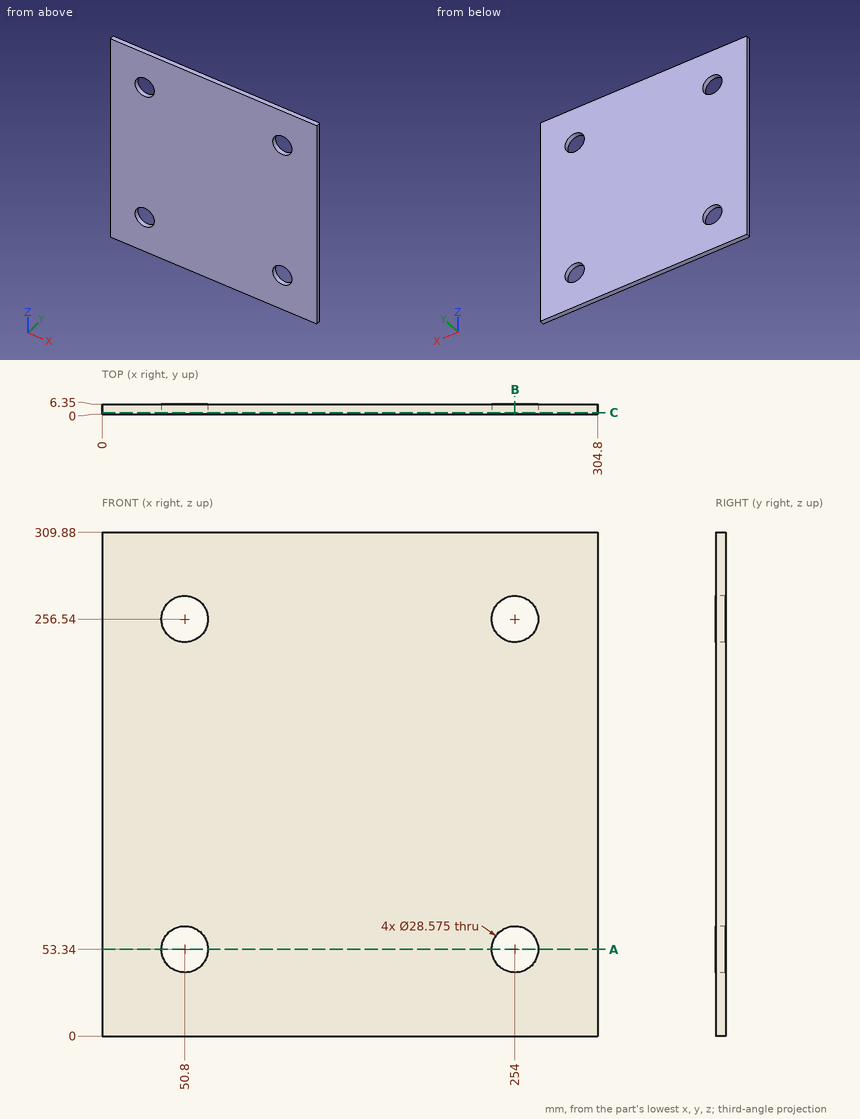
Job drawing, mm, ordinate dimensions from the low corner. One solid piece. Round coordinates to 2 decimals unless told otherwise and drop trailing zeros. Loops run counter-clockwise (first coordinate to the right, second up) from the corner with the lowest first, then second, coordinate; pieces in that order, holes last. Notation, with made-up numbers: M -16.75,41 L 15.25,41 A28 ccw 15.25,78 Z; hole C 27,44.25 d11. An arc over 180 degrees is marked long. Answer as CSV lines item,"result".
1. Cut at B-B on x = 254. Write the cut outline in (y, z), then the cut area to 3 significant figures.
Resolved:
outline,"M 0,0 L 6.35,0 L 6.35,39.05 L 0,39.05 Z; M 0,67.63 L 6.35,67.63 L 6.35,242.25 L 0,242.25 Z; M 0,270.83 L 6.35,270.83 L 6.35,309.88 L 0,309.88 Z"
area,"1,600 mm²"
2. Cut at A-A on z = 53.34. Write the cut outline in (x, y).
Resolved:
outline,"M 0,0 L 36.51,0 L 36.51,6.35 L 0,6.35 Z; M 65.09,0 L 239.71,0 L 239.71,6.35 L 65.09,6.35 Z; M 268.29,0 L 304.8,0 L 304.8,6.35 L 268.29,6.35 Z"
3. Flat gauge pins, fed straight in: P1, Ø3, axis at x = 137, z = 182.5, coming from the -Y side; P2, Ø17, axis at x = 50.8, z = 53.34, coming from the +Y side. Where does each tip first touch, or does it go through?
Resolved:
P1,"stops at y = 0"
P2,"passes through"
4. Cut at C-C on y = 1. Write the cut outline in (x, z) (1 decimal), then the cut area to 3 significant figures.
Resolved:
outline,"M 0,0 L 304.8,0 L 304.8,309.9 L 0,309.9 Z; hole C 50.8,53.3 d28.6; hole C 50.8,256.5 d28.6; hole C 254,53.3 d28.6; hole C 254,256.5 d28.6"
area,"91,900 mm²"
5. Wall check: probe 1 along X at (y, z) = (3.75, 256.54); probe 2 along Z at (x, y) = (254, 2); probe 3 along X at (y, z) = (2, 255). Give the ranges that are in metal, low to high. Write a range as [from, to].
Resolved:
probe 1,"x = [0, 36.51], [65.09, 239.71], [268.29, 304.8]"
probe 2,"z = [0, 39.05], [67.63, 242.25], [270.83, 309.88]"
probe 3,"x = [0, 36.6], [65, 239.8], [268.2, 304.8]"
